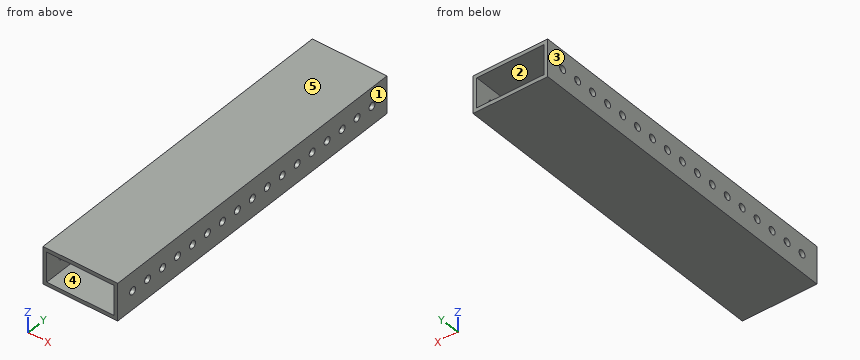
from build123d import *

# Parameters (mm, degrees)
SKETCH1_W           = 50.8
SKETCH1_H           = 25.4
SKETCH1_W_2         = 45.72
SKETCH1_H_2         = 20.32
BOSS_EXTRUDE1_DEPTH = 228.6
SKETCH2_R           = 2.54
CUT_EXTRUDE1_DEPTH  = 228.6


with BuildPart() as part:
    # Sketch1 → Boss-Extrude1 (new body)
    with BuildSketch(Plane(origin=(0, 0, 0), x_dir=(1, 0, 0), z_dir=(0, 1, 0))):
        with Locations((-4.028965517, 7.663793103)):
            Rectangle(SKETCH1_W, SKETCH1_H)
        with Locations((-4.028965517, 7.663793103)):
            Rectangle(SKETCH1_W_2, SKETCH1_H_2, mode=Mode.SUBTRACT)
    extrude(amount=BOSS_EXTRUDE1_DEPTH)

    # Sketch2 → Cut-Extrude1 (cut)
    with BuildSketch(Plane(origin=(21.371034483, 0, 0), x_dir=(0, 0, -1), z_dir=(1, 0, 0))):
        with Locations((7.663793103, 215.9)):
            Circle(SKETCH2_R)
        with Locations((7.663793103, 203.2)):
            Circle(SKETCH2_R)
        with Locations((7.663793103, 190.5)):
            Circle(SKETCH2_R)
        with Locations((7.663793103, 177.8)):
            Circle(SKETCH2_R)
        with Locations((7.663793103, 165.1)):
            Circle(SKETCH2_R)
        with Locations((7.663793103, 152.4)):
            Circle(SKETCH2_R)
        with Locations((7.663793103, 139.7)):
            Circle(SKETCH2_R)
        with Locations((7.663793103, 127)):
            Circle(SKETCH2_R)
        with Locations((7.663793103, 114.3)):
            Circle(SKETCH2_R)
        with Locations((7.663793103, 101.6)):
            Circle(SKETCH2_R)
        with Locations((7.663793103, 88.9)):
            Circle(SKETCH2_R)
        with Locations((7.663793103, 76.2)):
            Circle(SKETCH2_R)
        with Locations((7.663793103, 63.5)):
            Circle(SKETCH2_R)
        with Locations((7.663793103, 50.8)):
            Circle(SKETCH2_R)
        with Locations((7.663793103, 38.1)):
            Circle(SKETCH2_R)
        with Locations((7.663793103, 25.4)):
            Circle(SKETCH2_R)
        with Locations((7.663793103, 12.7)):
            Circle(SKETCH2_R)
    extrude(amount=-CUT_EXTRUDE1_DEPTH, mode=Mode.SUBTRACT)


solid = part.part
Model file for the job. Use its own axes, mm. Face numbers are marked on the shaded views. A direction names the side the tool comes from. Give positions to 0.01 mm unless a question says otherwise; leave off trailing zeros. Write each loop counter-clockwise with the first axis right and the second up, starting at its lowest first coordinate (ties: lowest second). Pieces come first, ordered by that corner, then holes. Notation, with made-up numbers: (67, -9) -> (114, -9) arc R25 ccw to (114, 22) -> close; hole circle Ø9 at (77.5, 51). An arc over 180 degrees is marked (long way). Write item = value, one per line.
(1) Slice it at B-B, the plane y = 88.9. Give the cut face in (x, z), then the cut area to 3 significant figures.
Determined:
outline = (-29.43, -20.36) -> (21.37, -20.36) -> (21.37, -10.2) -> (18.83, -10.2) -> (18.83, -17.82) -> (-26.89, -17.82) -> (-26.89, -10.2) -> (-29.43, -10.2) -> close; (-29.43, -5.12) -> (-26.89, -5.12) -> (-26.89, 2.5) -> (18.83, 2.5) -> (18.83, -5.12) -> (21.37, -5.12) -> (21.37, 5.04) -> (-29.43, 5.04) -> close
area = 335 mm2
(2) Tool access for the marked faces 4 and 5: list every direction of +Z, -Z, +X, -X, +Y, -Y with a clear straight run to the whole face (end or side of a thin tool).
Determined:
face_4 = +Y, -Y
face_5 = +Z, +X, -X, +Y, -Y
(3) Mould opens along X. For the marked faces 1, 2 and 3 say: released by +X, released by -X, zero draft, split by the parting line, or undercut.
Determined:
face_1 = released by +X
face_2 = undercut
face_3 = released by -X
(4) Probe line 1 along X through (y, z) = (86, -2.75); line 2 along Z through (x, y) = (-28, 165); line 3 along Z through (x, y) = (-17.5, 30.5). List the from-to ranges inside material, lowest first.
Determined:
line_1 = -29.43 to -26.89, 18.83 to 21.37
line_2 = -20.36 to -10.2, -5.13 to 5.04
line_3 = -20.36 to -17.82, 2.5 to 5.04
(5) Slice it at C-C, the plane x = -6. Give the cut face in (y, z), then the cut area to 3 significant figures.
Determined:
outline = (0, -20.36) -> (228.6, -20.36) -> (228.6, -17.82) -> (0, -17.82) -> close; (0, 2.5) -> (228.6, 2.5) -> (228.6, 5.04) -> (0, 5.04) -> close
area = 1,160 mm2
(6) Slice it at A-A, the plane z = -1. Give the cut face in (x, y), then the cut area to 3 significant figures.
Determined:
outline = (-29.43, 0) -> (-26.89, 0) -> (-26.89, 228.6) -> (-29.43, 228.6) -> close; (18.83, 0) -> (21.37, 0) -> (21.37, 228.6) -> (18.83, 228.6) -> close
area = 1,160 mm2
(7) Slice it at D-D, the plane y = 20. Give the cut face in (x, z).
Determined:
outline = (-29.43, -20.36) -> (21.37, -20.36) -> (21.37, 5.04) -> (-29.43, 5.04) -> close; hole (-26.89, -17.82) -> (18.83, -17.82) -> (18.83, 2.5) -> (-26.89, 2.5) -> close
(8) Flat gauge pin, fed straight in: P1, Ø4, axis at y = 12.7, z = -7.66, coming from the -X side. Where does the tip first touch, or does it go through?
Determined:
P1 = through
